Source: three-view drawing plus pictorial views. Frame: mm from the lowest corner of the part. A direction names the side the tool comes from. Round coordinates to 2 decimals unless told otherwise and drop trailing zeros. Order: outer loops, then holes, each group sorted by start corner. A loop starts at its lowest first (then second) coordinate and runs counter-clockwise, first axis right, second up. Notation, with made-up numbers: (16, 84) -> (34, 84) arc R16 ccw to (34, 97) -> close; hole circle Ø7 at (68.25, 24.5). An arc over 180 degrees is marked (long way). Answer as CSV lines item,"result". Start each with the question number.
1) First-contact query: P1, Ø1.5, axis at x = 4, y = 10.5, coming from the +Z side. Flat tip, straight axial feed; report the tip coordinate or a pass-through.
2) Section query C-C, the plane y = 12.25. Output: boundary loops of the cut face in (x, z).
3) Access query for the marked faces 1 and 2. Directions: +Z, -Z, +X, -X, +Y, -Y. A direction counts if a zero-diameter tool reaches every point of the face in a straight line with its end or side. Return the directions, or none.
4) Line query: L1, parallel to X at y = 14.75, z = 5; L2, parallel to Y at x = 5.25, z = 0.75. Output: solid intervals per line, ascending.
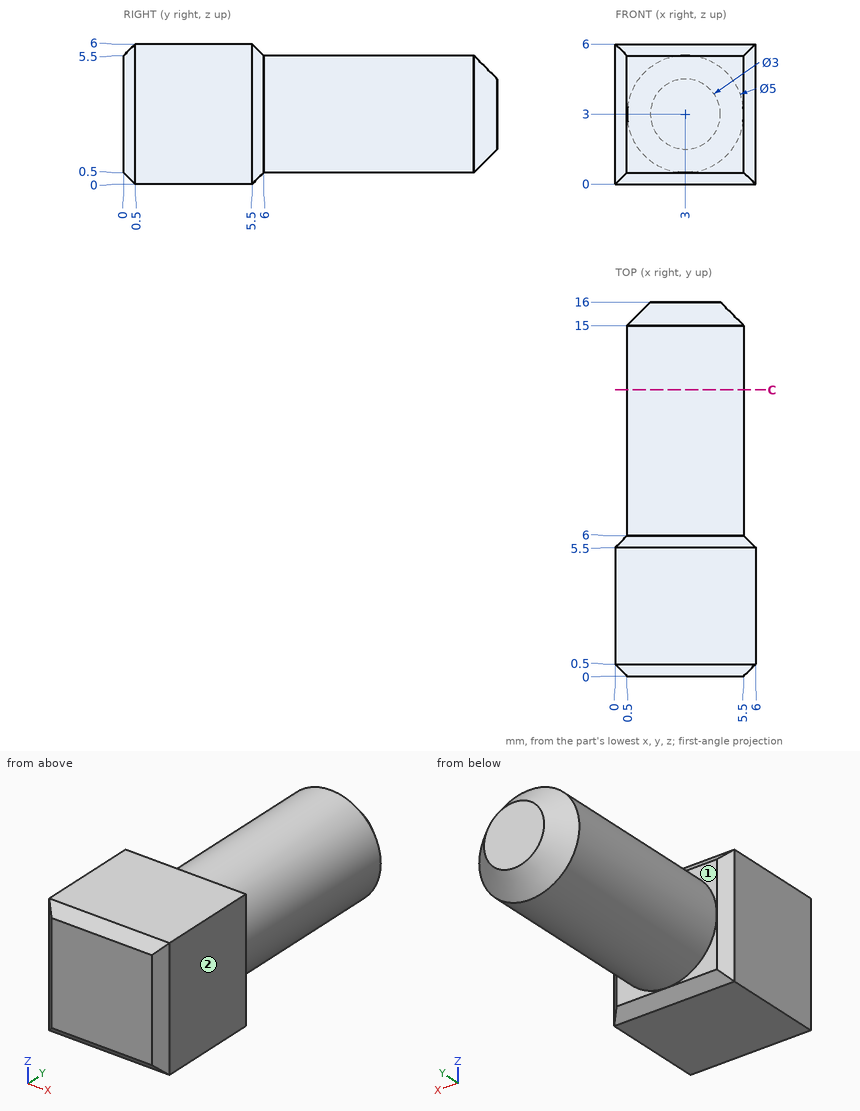
Findings:
1,P1,"stops at z = 5.49"
2,outline,"circle Ø5 at (3, 3)"
3,face 1,"+Y"
3,face 2,"+Z, -Z, +X, +Y, -Y"
4,L1,"x = 1.5 to 4.5"
4,L2,"y = 0 to 6"
